Could you check a few things on this model? Use its own coordinates, in mm. Face numbers are marked on the shaded views. Coordinates: 2 decimals unless noted, no trailing zeros. Write each loop counter-clockwise with the first axis right and the second up, starting at its lowest first coordinate (ties: lowest second). Pieces come first, ordered by that corner, then holes. Notation, with made-up numbers: M 45,75.5 L 88,75.5 A22 ccw 88,112.5 Z; hole C 70,68 d1. An arc over 180 degrees is marked long. Write item = value, one per line.
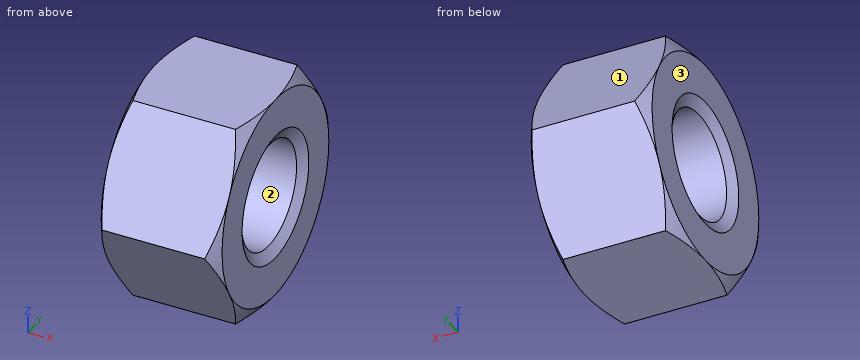
Autodesk Inventor part; units mm, degrees
ref_plane "Work Plane1" through (-8.3929, 0, 0) normal (0, -0.866, -0.5) x (1, 0, 0)
ref_plane "YZ Plane" through (0, 0, 0) normal (1, 0, 0) x (0, 1, 0)
ref_plane "XZ Plane" through (0, 0, 0) normal (0, 1, 0) x (-1, 0, 0)
sketch "Sketch1" plane through (0, 0, 0) normal (1, 0, 0) x (0, 1, 0)
  line L0 (-4.6188, 0) -> (-2.3094, 4)
  line L1 (-2.3094, 4) -> (2.3094, 4)
  line L2 (2.3094, 4) -> (4.6188, 0)
  line L3 (4.6188, 0) -> (2.3094, -4)
  line L4 (2.3094, -4) -> (-2.3094, -4)
  line L5 (-2.3094, -4) -> (-4.6188, 0)
  point P0 (0, 0)
  point P1 (0, 0)
  dimension "d0" = 9.2376
extrude "Body" add sketch "Sketch1" along normal blind 4.7
sketch "Sketch2" plane through (0, 0, 0) normal (0, 0, 1) x (1, 0, 0)
  line L0 (0, 2.3094) -> (0, 4.6188)
  line L1 (0, 4.6188) -> (4.7, 4.6188)
  line L2 (4.7, 2.3094) -> (4.7, 4.6188)
  line L3 (-0.94, 0) -> (5.64, 0)
  line L4 (0.3573, 4.6188) -> (0, 4)
  line L5 (4.3427, 4.6188) -> (4.7, 4)
  dimension "d3" = 30
  dimension "d4" = 30
  dimension "d5" = 8
  dimension "d6" = 8
revolve "Chamfer1" cut sketch "Sketch2" angle 360 about axis through (-10, 0, 0) along (1, 0, 0)
sketch "Sketch3" plane through (4.7, 0, 0) normal (1, 0, 0) x (0, 0, -1)
  arc A0 (-2, -3.4641) -> (2, -3.4641) centre (0, 0) ccw
hole "Thread" at (4.7, 0, 0) direction (-1, 0, 0) diameter 4.134 end through all
chamfer "Chamfer2" distance 0.433 angle 30 1 edges at (4.7, 0, 2.067) measured on face at (4.7, 3.336, -0.083)
chamfer "Chamfer3" distance 0.433 angle 30 1 edges at (0, 0, 2.067) measured on face at (0, 3.336, -0.083)
ref_plane "Work Plane1" through (-8.3929, 0, 0) normal (0, -0.866, -0.5) x (1, 0, 0)
equation "\"d0\" = 1.1547 * SW"
equation "\"d1\" = KOH"
equation "\"d3\" = ANG1"
equation "\"d4\" = ANG2"
equation "\"d5\" = SW0"
equation "\"d6\" = SW01"
equation "\"d8\" = -0.5 * GD1 + 0.5 * NND"
equation "\"d40\" = -0.5 * GD1 + 0.5 * NND"
equation "\"d10\" = -0.5 * GD1 + 0.5 * NND"
equation "\"d41\" = -0.5 * GD1 + 0.5 * NND"
equation "\"ANG1\" = 30deg"
equation "\"ANG2\" = 30deg"
equation "\"NND\" = 5"
equation "\"KOH\" = 4.7"
equation "\"SW\" = 8"
equation "\"SW0\" = SW"
equation "\"SW01\" = SW"
equation "\"GUL\" = 0.541266 * PTC"
equation "\"WFT\" = 0.5"
equation "\"THREADDIA\" = 5"
equation "\"TOA\" = 30deg"
equation "\"PTC\" = 0.8"
equation "\"E0\" = 1.155 * SW"
equation "\"GAL\" = 0.541266 * PTC"
properties part number "AS 1112 - M5  Type 5" material "Steel, Mild"
Item 1: Imagine slicing it at A-A (x = 3.3). Write out the boundary of the cut face in (y, z).
Numbers:
outline = M -4.62,0 L -2.31,-4 L 2.31,-4 L 4.62,0 L 2.31,4 L -2.31,4 Z; hole C 0,0 d4.13
Item 2: If I drill on line 1 along Z through (x, y) = (2.5, 0); line 2 along Y through (x, z) = (3.1, -1.75); line 3 along Y through (x, z) = (0.45, -0.5), over which ranges is the centre line in solid material (lowest first)?
Numbers:
line_1 = -4 to -2.07, 2.07 to 4
line_2 = -3.61 to -1.1, 1.1 to 3.61
line_3 = -4.33 to -2.01, 2.01 to 4.33
Item 3: I'm going to push flat-ended pins straight in: P1, Ø1.5, axis at y = 1.5, z = 0, coming from the +X side; P2, Ø2, axis at y = -1.5, z = 1, coming from the +X side. Where does each tip first touch, or does it pass through?
Numbers:
P1 = 4.56
P2 = 4.7
Item 4: If we mould it in two halves opening along Z, with no side actions, what happens to the marked faces 1, 2 and 3? For each: pulls with the +Z half, pulls with the -Z half, needs draft (parallel to the pull), parting line crosses it, or undercut.
Numbers:
face_1 = pulls with the +Z half
face_2 = undercut
face_3 = needs draft
